Geometry check sheet. Reference: the model listing, model coordinates, mm. Face numbers are marked on the shaded views. A direction names the side the tool comes from. Round coordinates to 2 decimals unless told otherwise and drop trailing zeros. Write each loop counter-clockwise with the first axis right and the second up, starting at its lowest first coordinate (ties: lowest second). Pieces come first, ordered by that corner, then holes. Notation, with made-up numbers: M 50.5,42 L 71.5,42 A19 cw 71.5,70 Z; hole C 7,-2 d6. An arc over 180 degrees is marked long. Put each result on its own line as item: value. Start each with the question number.
(1) Section check D-D on z = 6.75. Record the cut outline in (x, y).
(2) Tool access check on the marked faces 1, 2, 3, 4 and 5. Record the directions out of +Z, -Z, +X, -X, +Y, -Y that give a thin tool (end or side, any length) a straight path to the whole face; none if there is none.
(3) Section check C-C on z = 4.5. Record the cut outline in (x, y), then the cut area to 3 significant figures.
(4) Section check B-B on x = 0. Count the separate pieces of the cut face and the enclosed holes in it, then the cut area to 3 significant figures.
(5) Mould release check, pull along X, two halves, no side actions. Record for the marked faces 6, 7, 8 and 9: pulls with the +X half, pulls with the -X half, needs draft (parallel to the pull), parting line crosses it, or undercut.
(6) Gauge pin test, flat ends, axial feed: pin 1 (1.5 mm diameter, centred on x = 0, z = 7, fed in from +Y); pin 2 (2.5 mm diameter, centred on x = -11, z = 1, fed in from +Y); pin 3 (3 mm diameter, centred on y = -3.5, z = 5, fed in from -X); pin 4 (3 mm diameter, centred on y = 2.5, z = 8.5, fed in from +X). Record the tip position at first contact, or that the pin passes through.
(7) Material ranges on probe 1 along Y at (x, z) = (0, 8.35); probe 2 along Y at (x, z) = (-11, 1.2); probe 3 along X at (y, z) = (0.5, 7.25), recorded low to high.
(8) Section check A-A on y = -3.75. Record the cut outline in (x, z), then the cut area to 3 significant figures.
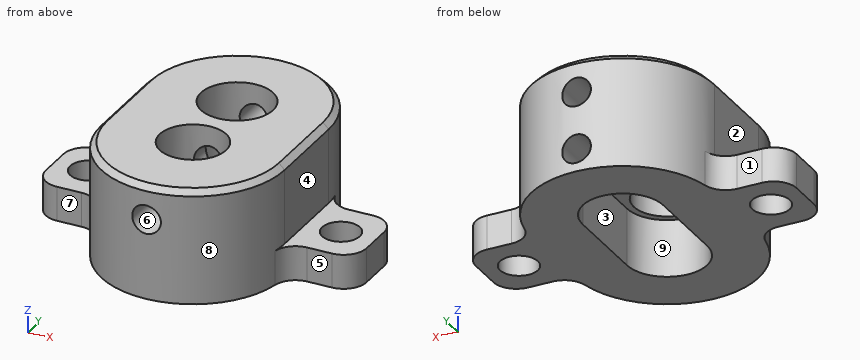
from build123d import *

# Parameters (mm, degrees)
SKETCH1_R            = 3.15
SKETCH1_R_2          = 2.9
BOSS_EXTRUDE1_DEPTH  = 10
SKETCH2_R            = 1.25
CUT_EXTRUDE1_DEPTH   = 21.105969263
CHAMFER1_SIZE        = 0.5
SKETCH3_R            = 1.25
CUT_EXTRUDE2_DEPTH   = 21.105969352
SKETCH4_W            = 6
SKETCH4_H            = 7
BOSS_EXTRUDE2_DEPTH  = 3
SKETCH5_R            = 1.65
CUT_EXTRUDE3_DEPTH   = 24.157072484
FILLET1_R            = 2
FILLET1_OF_MIRROR1_R = 2
FILLET2_R            = 2
CUT_EXTRUDE4_DEPTH   = 5


with BuildPart() as part:
    # Sketch1 → Boss-Extrude1 (new body)
    with BuildSketch(Plane.XY):
        with BuildLine():
            Line((8, 0), (8, -7.5))
            ThreePointArc((8, -7.5), (0, -15.5), (-8, -7.5))
            Line((-8, -7.5), (-8, 0))
            ThreePointArc((-8, 0), (0, 8), (8, 0))
        make_face()
        Circle(SKETCH1_R, mode=Mode.SUBTRACT)
        with Locations((0, -7.5)):
            Circle(SKETCH1_R_2, mode=Mode.SUBTRACT)
    extrude(amount=BOSS_EXTRUDE1_DEPTH)

    # Sketch2 → Cut-Extrude1 (cut, through all)
    with BuildSketch(Plane(origin=(0, 0, 0), x_dir=(1, 0, 0), z_dir=(0, 1, 0))):
        with Locations(Location((0, -2, 0), (0, 0, 90))):
            Circle(SKETCH2_R)
        with Locations(Location((0, -7, 0), (0, 0, 90))):
            Circle(SKETCH2_R)
    extrude(amount=CUT_EXTRUDE1_DEPTH, mode=Mode.SUBTRACT)

    # Chamfer1
    chamfer1_edges = [part.edges().sort_by_distance(p)[0] for p in [
        (0, -15.5, 10),
        (8, -3.75, 10),
        (0, 8, 10),
        (-8, -3.75, 10),
    ]]
    chamfer(chamfer1_edges, length=CHAMFER1_SIZE)

    # Sketch3 → Cut-Extrude2 (cut, through all)
    with BuildSketch(Plane(origin=(0, 0, 0), x_dir=(1, 0, 0), z_dir=(0, 1, 0))):
        with Locations(Location((0, -7, 0), (0, 0, 90))):
            Circle(SKETCH3_R)
    extrude(amount=-CUT_EXTRUDE2_DEPTH, mode=Mode.SUBTRACT)

    # Sketch4 → Boss-Extrude2 (add)
    with BuildSketch(Plane(origin=(0, 0, 0), x_dir=(-1, 0, 0), z_dir=(0, 0, -1))):
        with Locations((-11, -3.75)):
            Rectangle(SKETCH4_W, SKETCH4_H)
    boss_extrude2 = extrude(amount=-BOSS_EXTRUDE2_DEPTH)

    # Sketch5 → Cut-Extrude3 (cut, through all)
    with BuildSketch(Plane(origin=(0, 0, 0), x_dir=(-1, 0, 0), z_dir=(0, 0, -1))):
        with Locations((-11, -3.75)):
            Circle(SKETCH5_R)
    cut_extrude3 = extrude(amount=-CUT_EXTRUDE3_DEPTH, mode=Mode.SUBTRACT)

    # Fillet1
    fillet1_edges = [part.edges().sort_by_distance(p)[0] for p in [
        (14, -7.25, 1.5),
        (14, -0.25, 1.5),
    ]]
    fillet(fillet1_edges, radius=FILLET1_R)

    # Mirror1: Boss-Extrude2, Cut-Extrude3 across plane
    add(boss_extrude2.mirror(Plane(origin=(0, 0, 0), x_dir=(0, 0, 1), z_dir=(1, 0, 0))))
    add(cut_extrude3.mirror(Plane(origin=(0, 0, 0), x_dir=(0, 0, 1), z_dir=(1, 0, 0))), mode=Mode.SUBTRACT)

    # Fillet1 of Mirror1
    fillet1_of_mirror1_edges = [part.edges().sort_by_distance(p)[0] for p in [
        (-14, -7.25, 1.5),
        (-14, -0.25, 1.5),
    ]]
    fillet(fillet1_of_mirror1_edges, radius=FILLET1_OF_MIRROR1_R)

    # Fillet2
    # the kernel refuses this fillet: 2 mm, written as the material it adds along each edge
    with BuildSketch(Plane(origin=(-8, -0.25, 0), x_dir=(-1, 0, 0), z_dir=(0, 0, 1))) as fillet2_piece_1:
        with BuildLine():
            CenterArc((1.845684334, -2), FILLET2_R, 90, 79.921341892)
            Line((-0.123452533, -1.65), (-0.32036622, -1.615))
            ThreePointArc((-0.32036622, -1.615), (-0.2, -0.25), (-0.2, 0))
            Line((-0.2, 0), (0, 0.2))
            Line((0, 0.2), (1.845684334, 0.2))
            Line((1.845684334, 0.2), (1.845684334, 0))
        make_face()
    extrude(amount=3)
    with BuildSketch(Plane(origin=(-8, -7.25, 0), x_dir=(0.07461117211724091, -0.9972127019825267, 0), z_dir=(0, 0, 1)), Plane(origin=(8, -0.25, 0), x_dir=(-0.07461117211724083, 0.9972127019825267, 0), z_dir=(0, 0, 1))) as fillet2_piece_2:
        with BuildLine():
            CenterArc((1.856716732, -1.989762206), FILLET2_R, 95.799776596, 79.921341892)
            Line((-0.137708672, -1.840539861), (-0.337151212, -1.825617627))
            Line((-0.337151212, -1.825617627), (-0.19944254, 0.014922234))
            Line((-0.19944254, 0.014922234), (0.014922234, 0.19944254))
            ThreePointArc((0.014922234, 0.19944254), (0.26422541, 0.180789747), (1.634401413, 0.198976221))
            Line((1.634401413, 0.198976221), (1.654611896, 0))
        make_face()
    extrude(amount=3)
    with BuildSketch(Plane(origin=(8, -7.25, 0), x_dir=(-0.07461117211724076, -0.9972127019825267, 0), z_dir=(0, 0, 1))) as fillet2_piece_3:
        with BuildLine():
            CenterArc((1.856716732, 1.989762206), FILLET2_R, 184.278881512, 79.921341892)
            Line((-0.137708672, 1.840539861), (-0.337151212, 1.825617627))
            Line((-0.337151212, 1.825617627), (-0.19944254, -0.014922234))
            Line((-0.19944254, -0.014922234), (0.014922234, -0.19944254))
            ThreePointArc((0.014922234, -0.19944254), (0.26422541, -0.180789747), (1.634401413, -0.198976221))
            Line((1.634401413, -0.198976221), (1.654611896, 0))
        make_face()
    extrude(amount=3)

    # Sketch6 → Cut-Extrude4 (cut)
    with BuildSketch(Plane(origin=(0, 0, 0), x_dir=(-1, 0, 0), z_dir=(0, 0, -1))):
        with BuildLine():
            Line((3.5, 0), (3.5, -7.5))
            ThreePointArc((3.5, -7.5), (0, -11), (-3.5, -7.5))
            Line((-3.5, -7.5), (-3.5, 0))
            ThreePointArc((-3.5, 0), (0, 3.5), (3.5, 0))
        make_face()
    extrude(amount=-CUT_EXTRUDE4_DEPTH, mode=Mode.SUBTRACT)


solid = part.part
Answers follow:
1. outline: M -8,-7.5 A8 ccw -1.22,-15.41 L -1.22,-10.13 A2.9 cw -1.22,-4.87 L -1.22,-2.9 A3.15 cw -1.22,2.9 L -1.22,7.91 A8 ccw -8,0 Z; M 1.22,-15.41 A8 ccw 8,-7.5 L 8,0 A8 ccw 1.22,7.91 L 1.22,2.9 A3.15 cw 1.22,-2.9 L 1.22,-4.87 A2.9 cw 1.22,-10.13 Z
2. face 1: +Z, -Z, -X, +Y
2. face 2: +Z, -X, +Y, -Y
2. face 3: -Z
2. face 4: +Z, +X, +Y, -Y
2. face 5: +Z, -Z, +X, -Y
3. outline: M -8,-7.5 A8 ccw 8,-7.5 L 8,0 A8 ccw -8,0 Z; hole M -3.5,-7.5 A3.5 ccw 3.5,-7.5 L 3.5,0 A3.5 ccw -3.5,0 Z
3. area: 230 mm^2
4. separate pieces: 7
4. enclosed holes: 0
4. area: 62.0 mm^2
5. face 6: undercut
5. face 7: needs draft
5. face 8: parting line crosses it
5. face 9: undercut
6. pin 1: passes through
6. pin 2: stops at y = -0.25
6. pin 3: stops at x = -8
6. pin 4: stops at x = 7.94
7. probe 1: y = -15.5 to -10.4, -4.6 to -3.15, 3.15 to 8
7. probe 2: y = -7.25 to -5.4, -2.1 to -0.25
7. probe 3: x = -7.98 to -3.11, 3.11 to 7.98
8. outline: M -14,0 L -12.65,0 L -12.65,3 L -14,3 Z; M -9.35,0 L -3.5,0 L -3.5,5 L 3.5,5 L 3.5,0 L 9.35,0 L 9.35,3 L 8,3 L 8,9.5 L 7.5,10 L -7.5,10 L -8,9.5 L -8,3 L -9.35,3 Z; M 12.65,0 L 14,0 L 14,3 L 12.65,3 Z; hole C 0,7 d2.5
8. area: 136 mm^2
